Geometry: final body of the model. Coordinates: model frame, mm. A direction names the side the tool comes from. Coordinates: 2 decimals unless noted, no trailing zeros. Order: outer loops, then holes, each group sorted by start corner. A loop starts at its lowest first (then second) coordinate and runs counter-clockwise, first axis right, second up. Notation, with made-up numbers: (55.25, 49.25) - (100.25, 49.25) arc R17 ccw to (100.25, 68.25) - close; hole circle Ø7 at (49, -25). An arc over 180 degrees is marked (long way). Use one line per item in the form item = value. Start each with the question number.
```python
from build123d import *

# Parameters (mm, degrees)
SKETCH2_R          = 7
CUT_EXTRUDE1_DEPTH = 2.5
SKETCH3_R          = 2.1
CUT_EXTRUDE2_DEPTH = 6.5
SKETCH4_R          = 4
CUT_EXTRUDE3_DEPTH = 4.5
CUT_EXTRUDE4_REACH = 22
SKETCH5_W          = 4.2
SKETCH5_H          = 5.5
SKETCH5_H_2        = 3.449205174
SKETCH6_R          = 1
CUT_EXTRUDE5_DEPTH = 6.5000001


with BuildPart() as part:
    # Sketch1 → Revolve1 (revolve)
    with BuildSketch(Plane.XY):
        with BuildLine():
            Line((0, 0), (0, 8))
            Line((0, 8), (-8, 8))
            Line((-8, 8), (-8, 5.5))
            Line((-8, 5.5), (-10, 5.5))
            Line((-10, 5.5), (-10, 4))
            ThreePointArc((-10, 4), (-6.798437881, 2.876952648), (-5, 0))
            Line((-5, 0), (0, 0))
        make_face()
    revolve(axis=Axis((0, 0, 0), (0, 1, 0)))

    # Sketch2 → Cut-Extrude1 (cut)
    with BuildSketch(Plane(origin=(0, 8, 0), x_dir=(1, 0, 0), z_dir=(0, 1, 0))):
        Circle(SKETCH2_R)
    extrude(amount=-CUT_EXTRUDE1_DEPTH, mode=Mode.SUBTRACT)

    # Sketch3 → Cut-Extrude2 (cut, through all)
    with BuildSketch(Plane(origin=(0, 5.5, 0), x_dir=(1, 0, 0), z_dir=(0, 1, 0))):
        Circle(SKETCH3_R)
    extrude(amount=-CUT_EXTRUDE2_DEPTH, mode=Mode.SUBTRACT)

    # Sketch4 → Cut-Extrude3 (cut)
    with BuildSketch(Plane.XZ):
        Circle(SKETCH4_R)
    extrude(amount=-CUT_EXTRUDE3_DEPTH, mode=Mode.SUBTRACT)

    # Sketch5 → Cut-Extrude4 (cut, up to next)
    with BuildSketch(Plane.XY.offset(10), mode=Mode.PRIVATE) as cut_extrude4_sk1:
        with Locations((0, 2.75)):
            Rectangle(SKETCH5_W, SKETCH5_H)
    cut_extrude4_tool1 = extrude(cut_extrude4_sk1.sketch, amount=-CUT_EXTRUDE4_REACH, mode=Mode.PRIVATE) & part.part
    add(cut_extrude4_tool1.solids().sort_by_distance((0, 2.75, 10))[0], mode=Mode.SUBTRACT)
    # Sketch5 → Cut-Extrude4 (cut, up to next)
    with BuildSketch(Plane.XY.offset(10), mode=Mode.PRIVATE) as cut_extrude4_sk2:
        with Locations((0, 7.224602587)):
            Rectangle(SKETCH5_W, SKETCH5_H_2)
    cut_extrude4_tool2 = extrude(cut_extrude4_sk2.sketch, amount=-CUT_EXTRUDE4_REACH, mode=Mode.PRIVATE) & part.part
    add(cut_extrude4_tool2.solids().sort_by_distance((0, 7.224603, 10))[0], mode=Mode.SUBTRACT)

    # Sketch6 → Cut-Extrude5 (cut, through all)
    with BuildSketch(Plane(origin=(0, 5.5, 0), x_dir=(1, 0, 0), z_dir=(0, 1, 0))):
        with Locations((0, 5.5)):
            Circle(SKETCH6_R)
        with Locations((-4.763139721, 2.75)):
            Circle(SKETCH6_R)
        with Locations((-4.763139721, -2.75)):
            Circle(SKETCH6_R)
        with Locations((0, -5.5)):
            Circle(SKETCH6_R)
        with Locations((4.763139721, -2.75)):
            Circle(SKETCH6_R)
        with Locations((4.763139721, 2.75)):
            Circle(SKETCH6_R)
    extrude(amount=-CUT_EXTRUDE5_DEPTH, mode=Mode.SUBTRACT)


solid = part.part
```
(1) Cut plane B-B on x = 0. Return the cut outline in (y, z) (3 decimals), plus the area to 3 significant figures.
(2) Cut plane D-D on z = 2.75. Count the separate pieces of the cut face and the enclosed holes in it, plus the area to 3 significant figures.
(3) Set-up query: faces 1 (the cylindrical face through (-3.81, 3.4, 2.45)), 2 (the cylindrical face through (0, 7, -8)), 3 (the cylindrical face through (0, 2, -4)), 4 (the flat face through (-2.1, 4, 5)). Return all of +Z, -Z, +X, -X, +Y, -Y with unobstructed straight access to the full face (end or side cutting, diameter ignored); none if empty.
(4) Contact query for flat-ended pins moving along their axis: pin 1 Ø1.5 at (x, y) = (2, 1) entering from +Z; pin 2 Ø6 at (x, z) = (3, -1) entering from +Y; pin 3 Ø3 at (x, y) = (-6, 1.5) entering from -Z; pin 4 Ø1.6 at (x, z) = (4.76, 2.75) entering from -Y. Output: stop coordinate, or through.
(5) Draft query along Z for faces 5 (the cylindrical face through (0, 5, -2.1)), 6 (the cylindrical face through (3.97, 3.4, -2.14)), 7 (the flat face through (2.1, 4, 5)). Return one class per face: released by +Z, released by -Z, zero draft, split by the parting line, or undercut.
(6) Cut plane C-C on y = 7. Return the cut outline in (x, z).
(7) Material intervals for L1, parallel to Z at x = 4.75, y = 2.75; L2, parallel to X at y = 2.8, z = -2.75; L3, parallel to Z at x = -5, y = 5, sorted ascending. Write a range as from..to.
(8) Cut plane A-A on y = 5.25. Return the cut outline in (x, z).
Check sheet entries:
q1.outline = (0, -4.5) - (5.5, -4.5) - (5.5, -2.1) - (4.5, -2.1) - (4.5, -4) - (0, -4) - close; (2.619, -6.5) arc R5.125 cw to (4, -10) - (5.5, -10) - (5.5, -8) - (8, -8) - (8, -7) - (5.5, -7) - (5.5, -6.5) - close
q1.area = 13.9 mm^2
q2.separate_pieces = 4
q2.enclosed_holes = 0
q2.area = 31.6 mm^2
q3.face_1 = +Y, -Y
q3.face_2 = +Y
q3.face_3 = -Y
q3.face_4 = +Z, +Y, -Y
q4.pin_1 = 5.36
q4.pin_2 = 5.5
q4.pin_3 = -4.18
q4.pin_4 = through
q5.face_5 = released by +Z
q5.face_6 = undercut
q5.face_7 = zero draft
q6.outline = (-2.1, 6.68) - (-2.1, 7.72) arc R8 ccw (long way) to (2.1, 7.72) - (2.1, 6.68) arc R7 cw (long way) to start
q7.L1 = -4.65..-3.75, -1.75..1.75, 3.75..4.65
q7.L2 = -6.11..-5.76, -3.76..-2.9, 2.9..3.76, 5.76..6.11
q7.L3 = -8.66..-3.72, -1.78..1.78, 3.72..8.66
q8.outline = (-2.1, 0) - (-2.1, 9.78) arc R10 ccw (long way) to (2.1, 9.78) - (2.1, 0) arc R2.1 cw to start; hole circle Ø2 at (-4.76, -2.75); hole circle Ø2 at (-4.76, 2.75); hole circle Ø2 at (0, -5.5); hole circle Ø2 at (4.76, -2.75); hole circle Ø2 at (4.76, 2.75)
